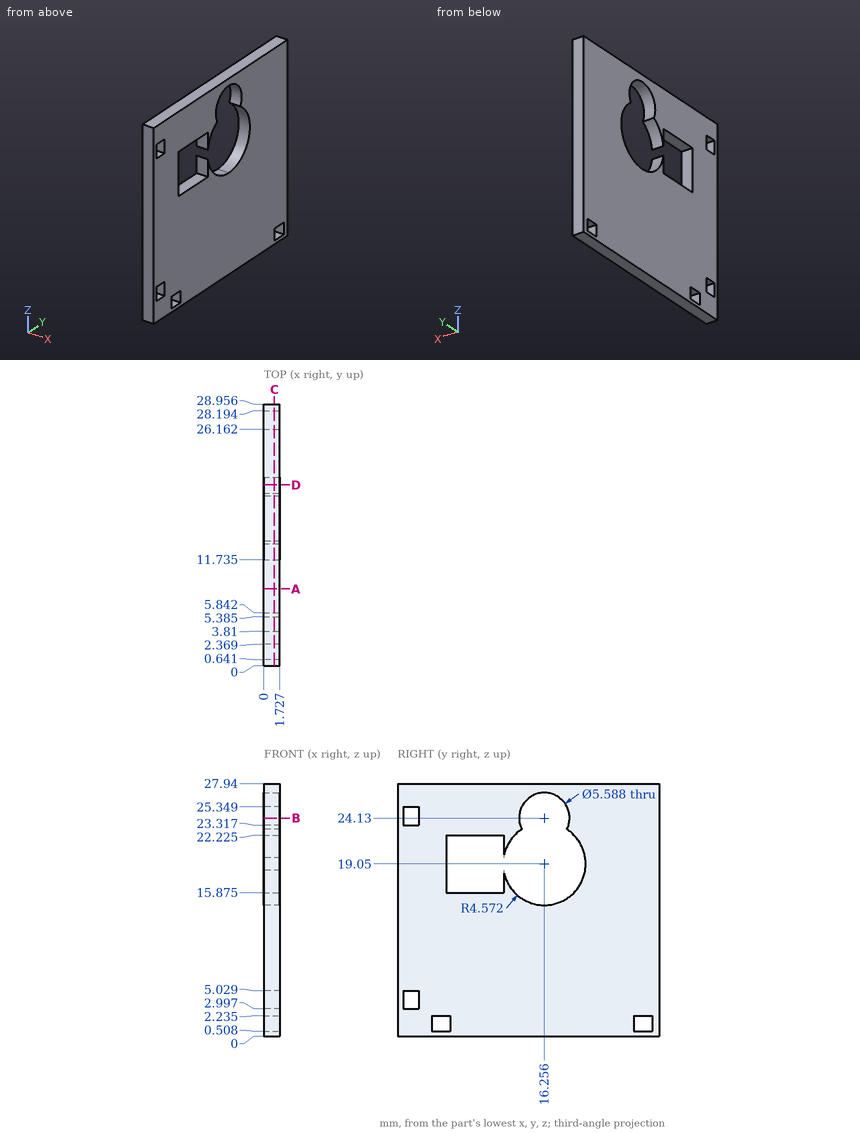
Here's the drawing with two shaded views (mm, measured from the low corner). I have some questions. Coordinates: 2 decimals unless noted, no trailing zeros. Order: outer loops, then holes, each group sorted by start corner. A loop starts at its lowest first (then second) coordinate and runs counter-clockwise, first axis right, second up. Notation, with made-up numbers: (81, -16) - (128, -16) arc R21 ccw to (128, 5) - close; hole circle Ø3 at (-26.75, -33.5). An arc over 180 degrees is marked (long way). Use CSV: the item, a comma, the result in double quotes. Start each with the question number.
1. Please list where these lines run through material, in increasing order: line 1 (Y direction, x = 0.9, z = 24.13); line 2 (Z direction, x = 0.65, y = 5.75) (1 decimal); line 3 (Y direction, x = 0.9, z = 19) (1 decimal). Write a range as from..to.
2. Suppose I cut it at C-C on x = 1.15. Give the number of separate pieces and of enclosed holes in the cut face.
3. Suppose I cut it at D-D on y = 20. List the corners of the cut face in (x, z) for me.
4. Suppose I cut it at A-A on y = 8.5. List the corners of the cut face in (x, z) for me (1 decimal).
5. Suppose I cut it at B-B on z = 24.13. List the corners of the cut face in (x, y) for me.
Output:
1,line 1,"y = 0..0.64, 2.37..13.46, 19.05..28.96"
1,line 2,"z = 0..0.5, 2.2..15.9, 22.2..27.9"
1,line 3,"y = 0..5.4, 20.8..29"
2,separate pieces,"1"
2,enclosed holes,"5"
3,outline,"(0, 0) - (1.73, 0) - (1.73, 16.43) - (0, 16.43) - close; (0, 21.67) - (1.73, 21.67) - (1.73, 27.94) - (0, 27.94) - close"
4,outline,"(0, 0) - (1.7, 0) - (1.7, 15.9) - (0, 15.9) - close; (0, 22.2) - (1.7, 22.2) - (1.7, 27.9) - (0, 27.9) - close"
5,outline,"(0, 0) - (1.73, 0) - (1.73, 0.64) - (0, 0.64) - close; (0, 2.37) - (1.73, 2.37) - (1.73, 13.46) - (0, 13.46) - close; (0, 19.05) - (1.73, 19.05) - (1.73, 28.96) - (0, 28.96) - close"
